For this review, take the finished solid that the model builds, in its own axes (mm). A direction names the side the tool comes from. Coordinates: 2 decimals unless noted, no trailing zeros. Loops run counter-clockwise (first coordinate to the right, second up) from the corner with the lowest first, then second, coordinate; pieces in that order, holes last.
1. Clearance check with flat-ended pins moving along their axes: P1, Ø2, axis at x = 65, y = -16.5, coming from the +Z side; P2, Ø0.8, axis at x = 65, z = 0.5, coming from the -Y side; P3, Ø2, axis at x = 65, y = -11.5, coming from the +Z side. State where each tip first meets the part, or that it passes through.
2. Mouldability with a two-part tool opening along Z and no side actions: class faces 1 (the face through (-4.493, 5.586, -3.562)), 2 (the face through (64.72, 0.377, 20.296)), 3 (the face through (4.83, -20.65, -4.58)), 4 (the face through (75.2, 0, 0)) as pulls with the +Z half, pulls with the -Z half, needs draft (parallel to the pull), parting line crosses it, or undercut.
3. Take a section at A-A, the plane x = 57. State the section outline as (y, z) points, then the cut area to 3 significant figures.
4. Take a section at B-B, the plane x = 39.5. State the section outline as (y, z) points.
5. Machinability: for faces 5 (the face through (69, -17.5, 0)), 6 (the face through (5.831, 15.615, 1.216)), 7 (the face through (65, -18, 4.875)), which of the approach directions +Z, -Z, +X, -X, +Y, -Y give a long, thin tool a straight path to every point of the face, cutting with its end or side? Answer none if there is none.
6. To check wall thickness, follow probe 1 along Y at (x, z) = (72, 0); probe 2 along Y at (x, z) = (8.5, 1); probe 3 along Z at (x, y) = (5, -8). State the ranges of each line that lie inside material, in increasing order.
```python
from build123d import *

# Parameters (mm, degrees)
SKETCH1_W                   = 34
SKETCH1_H                   = 22.15
SKETCH2_R                   = 21.15
BOSS_EXTRUDE1_DEPTH         = 25
SKETCH3_W                   = 4.6
SKETCH3_H                   = 0.5
BOSS_EXTRUDE2_DEPTH         = 8.15
CUT_EXTRUDE1_DEPTH          = 40.65
SKETCH5_W                   = 4.6
SKETCH5_H                   = 0.5
BOSS_EXTRUDE3_DEPTH         = 8.15
CUT_EXTRUDE2_REACH          = 41.65
CUT_EXTRUDE3_DEPTH          = 2.8
SKETCH8_R                   = 14.25
BOSS_EXTRUDE4_DEPTH         = 1
CUT_EXTRUDE4_DEPTH          = 2
CUT_EXTRUDE5_DEPTH          = 2
CUT_EXTRUDE6_DEPTH          = 2
CUT_EXTRUDE7_DEPTH          = 2
SKETCH13_R                  = 21.15
BOSS_EXTRUDE5_DEPTH         = 7.1
CUT_EXTRUDE8_DEPTH          = 10
CUT_EXTRUDE9_DEPTH          = 10
CUT_EXTRUDE10_DEPTH         = 10
CUT_EXTRUDE11_DEPTH         = 10
SKETCH18_R                  = 8.75
BOSS_EXTRUDE6_DEPTH         = 8.5
HOLE1_D                     = 8
HOLE1_DEPTH                 = 1
SKETCH21_R                  = 8.9
BOSS_EXTRUDE7_DEPTH         = 5
F_1_2_CLEARANCE_HOLE1_D     = 13.25
F_1_2_CLEARANCE_HOLE1_DEPTH = 1
SKETCH25_W                  = 3.4
SKETCH25_H                  = 2.5
F_2_CLEARANCE_HOLE1_D       = 2.5
F_2_CLEARANCE_HOLE1_DEPTH   = 0.1
F_4_CLEARANCE_HOLE1_D       = 3.3
F_4_CLEARANCE_HOLE1_DEPTH   = 11.5
F_4_CLEARANCE_HOLE1_TIP     = 0.991420021
CHAMFER1_SIZE               = 0.5
FILLET1_R                   = 0.25
FILLET2_R                   = 0.75
FILLET3_R                   = 1
FILLET4_R                   = 2.5


with BuildPart() as part:
    # Sketch1 → Revolve1 (revolve)
    with BuildSketch(Plane.XY):
        with Locations((24.1, 11.075)):
            Rectangle(SKETCH1_W, SKETCH1_H)
    revolve(axis=Axis((7.1, 0, 0), (1, 0, 0)))

    # Sketch2 → Boss-Extrude1 (add)
    with BuildSketch(Plane(origin=(41.1, 0, 0), x_dir=(0, 0, -1), z_dir=(1, 0, 0))):
        Circle(SKETCH2_R)
    extrude(amount=BOSS_EXTRUDE1_DEPTH)

    # Sketch3 → Boss-Extrude2 (add)
    with BuildSketch(Plane(origin=(66.1, 0, 0), x_dir=(0, 0, -1), z_dir=(1, 0, 0))):
        with Locations((0, 17.25)):
            Rectangle(SKETCH3_W, SKETCH3_H)
    extrude(amount=BOSS_EXTRUDE2_DEPTH)

    # Sketch4 → Cut-Extrude1 (cut, through all)
    with BuildSketch(Plane(origin=(0, 17.5, 0), x_dir=(-1, 0, 0), z_dir=(0, 1, 0))):
        with BuildLine():
            Line((-71.25, -1), (-70.25, -1))
            ThreePointArc((-70.25, -1), (-69.25, 0), (-70.25, 1))
            Line((-70.25, 1), (-71.25, 1))
            ThreePointArc((-71.25, 1), (-72.25, 0), (-71.25, -1))
        make_face()
    extrude(amount=-CUT_EXTRUDE1_DEPTH, mode=Mode.SUBTRACT)

    # Sketch5 → Boss-Extrude3 (add)
    with BuildSketch(Plane(origin=(66.1, 0, 0), x_dir=(0, 0, -1), z_dir=(1, 0, 0))):
        with Locations((0, -17.25)):
            Rectangle(SKETCH5_W, SKETCH5_H)
    extrude(amount=BOSS_EXTRUDE3_DEPTH)

    # Sketch6 → Cut-Extrude2 (cut, up to next)
    with BuildSketch(Plane.XZ.offset(17.5), mode=Mode.PRIVATE) as cut_extrude2_sk1:
        with BuildLine():
            Line((71.25, 1), (70.25, 1))
            ThreePointArc((70.25, 1), (69.25, 0), (70.25, -1))
            Line((70.25, -1), (71.25, -1))
            ThreePointArc((71.25, -1), (72.25, 0), (71.25, 1))
        make_face()
    cut_extrude2_tool1 = extrude(cut_extrude2_sk1.sketch, amount=-CUT_EXTRUDE2_REACH, mode=Mode.PRIVATE) & part.part
    add(cut_extrude2_tool1.solids().sort_by_distance((70.75, -17.5, 0))[0], mode=Mode.SUBTRACT)

    # Sketch7 → Cut-Extrude3 (cut)
    with BuildSketch(Plane(origin=(66.1, 0, 0), x_dir=(0, 0, -1), z_dir=(1, 0, 0))):
        with BuildLine():
            Line((2.068879475, 14.25), (2.068879475, 15.25))
            Line((2.068879475, 15.25), (-4.875, 15.25))
            Line((-4.875, 15.25), (-4.875, 19.705947706))
            ThreePointArc((-4.875, 19.705947706), (-20.3, 0), (-4.875, -19.705947706))
            Line((-4.875, -19.705947706), (-4.875, -15.25))
            Line((-4.875, -15.25), (4.875, -15.25))
            Line((4.875, -15.25), (4.875, -19.705947706))
            ThreePointArc((4.875, -19.705947706), (20.3, 0), (4.875, 19.705947706))
            Line((4.875, 19.705947706), (4.875, 14.25))
            Line((4.875, 14.25), (2.068879475, 14.25))
        make_face()
    extrude(amount=-CUT_EXTRUDE3_DEPTH, mode=Mode.SUBTRACT)

    # Sketch8 → Boss-Extrude4 (add)
    with BuildSketch(Plane(origin=(63.3, 0, 0), x_dir=(0, 0, -1), z_dir=(1, 0, 0))):
        Circle(SKETCH8_R)
    extrude(amount=BOSS_EXTRUDE4_DEPTH)

    # Sketch9 → Cut-Extrude4 (cut)
    with BuildSketch(Plane(origin=(64.3, 0, 0), x_dir=(0, 0, -1), z_dir=(1, 0, 0))):
        with BuildLine():
            ThreePointArc((-5.652173913, 11.706960752), (-9.192388155, 9.192388155), (-11.706960752, 5.652173913))
            ThreePointArc((-11.706960752, 5.652173913), (-11.008331502, 3.649196836), (-9.005354425, 4.347826087))
            ThreePointArc((-9.005354425, 4.347826087), (-7.071067812, 7.071067812), (-4.347826087, 9.005354425))
            ThreePointArc((-4.347826087, 9.005354425), (-3.649196836, 11.008331502), (-5.652173913, 11.706960752))
        make_face()
    extrude(amount=-CUT_EXTRUDE4_DEPTH, mode=Mode.SUBTRACT)

    # Sketch10 → Cut-Extrude5 (cut)
    with BuildSketch(Plane(origin=(64.3, 0, 0), x_dir=(0, 0, -1), z_dir=(1, 0, 0))):
        with BuildLine():
            ThreePointArc((11.706960752, 5.652173913), (9.192388155, 9.192388155), (5.652173913, 11.706960752))
            ThreePointArc((5.652173913, 11.706960752), (3.649196836, 11.008331502), (4.347826087, 9.005354425))
            ThreePointArc((4.347826087, 9.005354425), (7.071067812, 7.071067812), (9.005354425, 4.347826087))
            ThreePointArc((9.005354425, 4.347826087), (11.008331502, 3.649196836), (11.706960752, 5.652173913))
        make_face()
    extrude(amount=-CUT_EXTRUDE5_DEPTH, mode=Mode.SUBTRACT)

    # Sketch11 → Cut-Extrude6 (cut)
    with BuildSketch(Plane(origin=(64.3, 0, 0), x_dir=(0, 0, -1), z_dir=(1, 0, 0))):
        with BuildLine():
            ThreePointArc((5.652173913, -11.706960752), (9.192388155, -9.192388155), (11.706960752, -5.652173913))
            ThreePointArc((11.706960752, -5.652173913), (11.008331502, -3.649196836), (9.005354425, -4.347826087))
            ThreePointArc((9.005354425, -4.347826087), (7.071067812, -7.071067812), (4.347826087, -9.005354425))
            ThreePointArc((4.347826087, -9.005354425), (3.649196836, -11.008331502), (5.652173913, -11.706960752))
        make_face()
    extrude(amount=-CUT_EXTRUDE6_DEPTH, mode=Mode.SUBTRACT)

    # Sketch12 → Cut-Extrude7 (cut)
    with BuildSketch(Plane(origin=(64.3, 0, 0), x_dir=(0, 0, -1), z_dir=(1, 0, 0))):
        with BuildLine():
            ThreePointArc((-11.706960752, -5.652173913), (-9.192388155, -9.192388155), (-5.652173913, -11.706960752))
            ThreePointArc((-5.652173913, -11.706960752), (-3.649196836, -11.008331502), (-4.347826087, -9.005354425))
            ThreePointArc((-4.347826087, -9.005354425), (-7.071067812, -7.071067812), (-9.005354425, -4.347826087))
            ThreePointArc((-9.005354425, -4.347826087), (-11.008331502, -3.649196836), (-11.706960752, -5.652173913))
        make_face()
    extrude(amount=-CUT_EXTRUDE7_DEPTH, mode=Mode.SUBTRACT)

    # Sketch13 → Boss-Extrude5 (add)
    with BuildSketch(Plane.ZY.offset(-7.1)):
        Circle(SKETCH13_R)
    extrude(amount=BOSS_EXTRUDE5_DEPTH)

    # Sketch14 → Cut-Extrude8 (cut)
    with BuildSketch(Plane.ZY):
        with BuildLine():
            Line((6.761892188, 14.500924593), (4.775586358, 10.241277994))
            ThreePointArc((4.775586358, 10.241277994), (7.990306627, 7.990306627), (10.241277994, 4.775586358))
            Line((10.241277994, 4.775586358), (14.500924593, 6.761892188))
            ThreePointArc((14.500924593, 6.761892188), (11.313708499, 11.313708499), (6.761892188, 14.500924593))
        make_face()
    extrude(amount=-CUT_EXTRUDE8_DEPTH, mode=Mode.SUBTRACT)

    # Sketch15 → Cut-Extrude9 (cut)
    with BuildSketch(Plane.ZY):
        with BuildLine():
            Line((-6.761892188, -14.500924593), (-4.775586358, -10.241277994))
            ThreePointArc((-4.775586358, -10.241277994), (-7.990306627, -7.990306627), (-10.241277994, -4.775586358))
            Line((-10.241277994, -4.775586358), (-14.500924593, -6.761892188))
            ThreePointArc((-14.500924593, -6.761892188), (-11.313708499, -11.313708499), (-6.761892188, -14.500924593))
        make_face()
    extrude(amount=-CUT_EXTRUDE9_DEPTH, mode=Mode.SUBTRACT)

    # Sketch16 → Cut-Extrude10 (cut)
    with BuildSketch(Plane.ZY):
        with BuildLine():
            Line((-14.500924593, 6.761892188), (-10.241277994, 4.775586358))
            ThreePointArc((-10.241277994, 4.775586358), (-7.990306627, 7.990306627), (-4.775586358, 10.241277994))
            Line((-4.775586358, 10.241277994), (-6.761892188, 14.500924593))
            ThreePointArc((-6.761892188, 14.500924593), (-11.313708499, 11.313708499), (-14.500924593, 6.761892188))
        make_face()
    extrude(amount=-CUT_EXTRUDE10_DEPTH, mode=Mode.SUBTRACT)

    # Sketch17 → Cut-Extrude11 (cut)
    with BuildSketch(Plane.ZY):
        with BuildLine():
            Line((14.500924593, -6.761892188), (10.241277994, -4.775586358))
            ThreePointArc((10.241277994, -4.775586358), (7.990306627, -7.990306627), (4.775586358, -10.241277994))
            Line((4.775586358, -10.241277994), (6.761892188, -14.500924593))
            ThreePointArc((6.761892188, -14.500924593), (11.313708499, -11.313708499), (14.500924593, -6.761892188))
        make_face()
    extrude(amount=-CUT_EXTRUDE11_DEPTH, mode=Mode.SUBTRACT)

    # Sketch18 → Boss-Extrude6 (add)
    with BuildSketch(Plane(origin=(64.3, 0, 0), x_dir=(0, 0, -1), z_dir=(1, 0, 0))):
        Circle(SKETCH18_R)
    extrude(amount=BOSS_EXTRUDE6_DEPTH)

    # Hole1
    with Locations(Plane(origin=(72.8, 0, 0), x_dir=(0, 0, -1), z_dir=(1, 0, 0))):
        with Locations((0, 0)):
            Hole(HOLE1_D / 2, depth=HOLE1_DEPTH)

    # Sketch21 → Boss-Extrude7 (add)
    with BuildSketch(Plane.ZY):
        Circle(SKETCH21_R)
    extrude(amount=BOSS_EXTRUDE7_DEPTH)

    # 1/2 Clearance Hole1
    with Locations(Plane.ZY.offset(5)):
        with Locations((0, 0)):
            Hole(F_1_2_CLEARANCE_HOLE1_D / 2, depth=F_1_2_CLEARANCE_HOLE1_DEPTH)

    # Sketch24 → Revolve2 (revolve)
    with BuildSketch(Plane(origin=(0, 0, 0), x_dir=(-1, 0, 0), z_dir=(0, 0, -1))):
        Polygon((4, 3.75), (4, 0), (12.8, 0), (12.8, 2.5), (5, 2.5), (5, 3.75), align=None)
    revolve(axis=Axis((-4, 0, 0), (-1, 0, 0)))

    # Sketch25 → Revolve3 (revolve)
    with BuildSketch(Plane(origin=(0, 0, 0), x_dir=(-1, 0, 0), z_dir=(0, 0, -1))):
        with Locations((-73.5, 1.25)):
            Rectangle(SKETCH25_W, SKETCH25_H)
    revolve(axis=Axis((75.2, 0, 0), (-1, 0, 0)))

    # #2 Clearance Hole1
    with Locations(Plane(origin=(63.3, 0, 0), x_dir=(0, 0, -1), z_dir=(1, 0, 0))):
        with Locations((6.5, 15)):
            Hole(F_2_CLEARANCE_HOLE1_D / 2, depth=F_2_CLEARANCE_HOLE1_DEPTH)

    # #4 Clearance Hole1
    with Locations(Plane.ZY):
        with Locations((0, 14.5), (0, -14.5)):
            Hole(F_4_CLEARANCE_HOLE1_D / 2, depth=F_4_CLEARANCE_HOLE1_DEPTH)
            with Locations((0, 0, -(F_4_CLEARANCE_HOLE1_DEPTH + F_4_CLEARANCE_HOLE1_TIP / 2))):  # 118° drill point
                Cone(0, F_4_CLEARANCE_HOLE1_D / 2, F_4_CLEARANCE_HOLE1_TIP, mode=Mode.SUBTRACT)

    # Chamfer1
    chamfer1_edges = [part.edges().sort_by_distance(p)[0] for p in [
        (74.25, 17.25, -2.3),
        (74.25, 17.25, 2.3),
        (74.25, -17.25, -2.3),
        (74.25, -17.25, 2.3),
    ]]
    chamfer(chamfer1_edges, length=CHAMFER1_SIZE)

    # Fillet1
    fillet1_edges = [part.edges().sort_by_distance(p)[0] for p in [
        (-12.8, -2.5, 0),
    ]]
    fillet(fillet1_edges, radius=FILLET1_R)

    # Fillet2
    fillet2_edges = [part.edges().sort_by_distance(p)[0] for p in [
        (-5, 0, -8.9),
    ]]
    fillet(fillet2_edges, radius=FILLET2_R)

    # Fillet3
    fillet3_edges = [part.edges().sort_by_distance(p)[0] for p in [
        (72.8, 0, 8.75),
    ]]
    fillet(fillet3_edges, radius=FILLET3_R)

    # Fillet4
    fillet4_edges = [part.edges().sort_by_distance(p)[0] for p in [
        (0, 0, -21.15),
    ]]
    fillet(fillet4_edges, radius=FILLET4_R)


solid = part.part
```
Results list:
1. P1: stops at z = 14.39
1. P2: stops at y = -21.15
1. P3: stops at z = 18.36
2. face 1: undercut
2. face 2: undercut
2. face 3: parting line crosses it
2. face 4: needs draft
3. outline: circle Ø42.3 at (0, 0)
3. area: 1,410 mm2
4. outline: circle Ø44.3 at (0, 0)
5. face 5: +Z, -Z, +X, -Y
5. face 6: -X
5. face 7: +X
6. probe 1: y = -8.73 to -4, -2.5 to 2.5, 4 to 8.73
6. probe 2: y = -22.13 to -15.81, -13.19 to 13.19, 15.81 to 22.13
6. probe 3: z = -19.58 to -13.86, -7.98 to 7.98, 13.86 to 19.58
